from build123d import *

# Parameters (mm, degrees)
SKETCH_6_R          = 4
EXTRUDE_2_DEPTH     = 7
M4X0_72_D           = 3.3
M4X0_72_DEPTH       = 9
M4X0_72_TIP         = 0.991420021
CUT_EXTRUDE_1_DEPTH = 7


with BuildPart() as part:
    # Эскиз1 → Повернуть1 (revolve)
    with BuildSketch(Plane(origin=(0, 0, 0), x_dir=(1, 0, 0), z_dir=(0, 1, 0))):
        Polygon((0, 9), (3.75, 9), (4, 0), (0, 0), align=None)
    revolve(axis=Axis((0, 0, 0), (0, 0, -1)))

    # Эскиз6 → Бобышка-Вытянуть2 (add)
    with BuildSketch(Plane.XY):
        Circle(SKETCH_6_R)
    extrude(amount=EXTRUDE_2_DEPTH)

    # Отверстие обработанное метчиком M4x0.72
    with Locations(Plane(origin=(0, 0, -9), x_dir=(-1, 0, 0), z_dir=(0, 0, -1))):
        with Locations((0, 0)):
            Hole(M4X0_72_D / 2, depth=M4X0_72_DEPTH)
            with Locations((0, 0, -(M4X0_72_DEPTH + M4X0_72_TIP / 2))):  # 118° drill point
                Cone(0, M4X0_72_D / 2, M4X0_72_TIP, mode=Mode.SUBTRACT)

    # Эскиз9 → Вырез-Вытянуть1 (cut)
    with BuildSketch(Plane.XY.offset(7)):
        with BuildLine():
            Line((-1.322875656, 1.5), (1.322875656, 1.5))
            ThreePointArc((1.322875656, 1.5), (0, -2), (-1.322875656, 1.5))
        make_face()
    extrude(amount=-CUT_EXTRUDE_1_DEPTH, mode=Mode.SUBTRACT)


solid = part.part
Geometry check sheet. Reference: the model listing, model coordinates, mm. A direction names the side the tool comes from. Coordinates: 2 decimals unless noted, no trailing zeros. Order: outer loops, then holes, each group sorted by start corner. A loop starts at its lowest first (then second) coordinate and runs counter-clockwise, first axis right, second up. Notation, with made-up numbers: (82.25, 89) -> (103.25, 89) arc R24 ccw to (103.25, 109) -> close; hole circle Ø8 at (35, 54.25). An arc over 180 degrees is marked (long way). Use a Markdown table: item, result. Add a question column.
1. Material ranges on L1, parallel to X at y = 0, z = 2; L2, parallel to X at y = 0, z = -6.5; L3, parallel to Y at x = 0, z = -6, recorded low to high.
2. Cross-section at B-B (y = 0). Enter the section's corners in (x, z).
3. Cross-section at A-A (x = 0). Enter the section's corners in (y, z), and give its area (3 significant figures).
4. Mould release check, pull along X, two halves, no side actions. Record for faces 1 (the face through (0, 2, 7)), 2 (the face through (0, 1.5, 4)), 3 (the face through (-0.84, 3.785, -4.437)): pulls with the +X half, pulls with the -X half, needs draft (parallel to the pull), parting line crosses it, or undercut.
5. Cross-section at C-C (z = 0.5). Enter the section's corners in (x, y), and give its area (3 significant figures).
6. Set-up check for faces 4 (the face through (-0.867, -3.905, 3.451)), 5 (the face through (0, -2, 4)): record each of +Z, -Z, +X, -X, +Y, -Y from which the full face is reachable in a straight line by a thin tool's end or side.
7. Cross-section at D-D (z = -5.75). Enter the section's corners in (x, y), and give its area (3 significant figures).
8. Go/stop test with flat-tipped pins: pin 1 Ø1.5 at (x, z) = (1, -6.5) entering from -Y; pin 2 Ø3 at (x, z) = (0.5, 4) entering from -Y; pin 3 Ø3 at (y, z) = (3, 2) entering from +X; pin 4 Ø2 at (x, z) = (0.5, -3.5) entering from +Y. Record where each tip stops, or that it passes through.
Filled sheet:
| question | item | result |
|---|---|---|
| 1 | L1 | -4 to -2, 2 to 4 |
| 1 | L2 | -3.82 to -1.65, 1.65 to 3.82 |
| 1 | L3 | -3.83 to -1.65, 1.65 to 3.83 |
| 2 | outline | (-4, 0) -> (-3.75, -9) -> (-1.65, -9) -> (-1.65, 0) -> (-2, 0) -> (-2, 7) -> (-4, 7) -> close; (1.65, -9) -> (3.75, -9) -> (4, 0) -> (4, 7) -> (2, 7) -> (2, 0) -> (1.65, 0) -> close |
| 3 | outline | (-4, 0) -> (-3.75, -9) -> (-1.65, -9) -> (-1.65, 0) -> (-2, 0) -> (-2, 7) -> (-4, 7) -> close; (1.5, 0.09) -> (1.65, 0) -> (1.65, -9) -> (3.75, -9) -> (4, 0) -> (4, 7) -> (1.5, 7) -> close |
| 3 | area | 71.5 mm2 |
| 4 | face 1 | needs draft |
| 4 | face 2 | undercut |
| 4 | face 3 | parting line crosses it |
| 5 | outline | circle Ø8 at (0, 0); hole (-1.32, 1.5) arc R2 ccw (long way) to (1.32, 1.5) -> close |
| 5 | area | 38.6 mm2 |
| 6 | face 4 | +Z, -Z |
| 6 | face 5 | +Z |
| 7 | outline | circle Ø7.68 at (0, 0); hole circle Ø3.3 at (0, 0) |
| 7 | area | 37.8 mm2 |
| 8 | pin 1 | y = -3.82 |
| 8 | pin 2 | y = -4 |
| 8 | pin 3 | x = 3.71 |
| 8 | pin 4 | y = 3.93 |
